Autodesk Inventor part; units mm, degrees
ref_plane "YZ Plane" through (0, 0, 0) normal (1, 0, 0) x (0, 1, 0)
ref_plane "XZ Plane" through (0, 0, 0) normal (0, 1, 0) x (-1, 0, 0)
ref_plane "XY Plane" through (0, 0, 0) normal (0, 0, 1) x (1, 0, 0)
ref_plane "Work Plane3" through (0, 0, 0) normal (0, 0, 1) x (1, 0, 0)
sketch "Sketch2" plane through (0, 0, 0) normal (0, 0, 1) x (1, 0, 0)
  arc A0 (-7.5753, -9.9544) -> (-9.0817, -9.6822) centre (-8, -8) ccw construction
  arc A1 (-9.9544, 7.5753) -> (-9.6822, 9.0817) centre (-8, 8) ccw construction
  line L0 (-8, 8) -> (-8, -8) construction
  line L1 (-3.2375, 8) -> (-3.2375, -8)
  line L2 (-12.7625, 8) -> (-12.7625, -3.2375)
  arc A2 (-3.2375, 8) -> (-12.7625, 8) centre (-8, 8) ccw
  arc A3 (-3.2375, 8) -> (-12.7625, 8) centre (-8, 8) ccw construction
  arc A4 (-8, -12.7625) -> (-3.2375, -8) centre (-8, -8) ccw
  line L3 (-76.8525, -130.4672) -> (11.0654, 135.3719) construction
  line L4 (-12.7625, -3.2375) -> (-34.7753, -3.2375)
  line L5 (-67.8092, -133.458) -> (20.1087, 132.3811) construction
  line L6 (-8, -12.7625) -> (-27.893, -12.7625)
  arc A5 (1.9836, 0.2558) -> (1.5702, -1.2387) centre (0, 0) ccw construction
  circle A6 centre (0, 0) radius 115.8748 construction
  line L7 (-34.7753, -3.2375) -> (-65.3505, -95.6884)
  line L8 (-65.3505, -95.6884) -> (-56.2232, -98.425)
  line L9 (-27.893, -12.7625) -> (-56.2232, -98.425)
  line L10 (-27.893, -12.7625) -> (-36.9363, -9.7717) construction
  line L11 (-60.7868, -97.0567) -> (-32.4146, -11.2671) construction
  circle A7 centre (-35.4852, -20.5515) radius 1.9685
  circle A8 centre (-38.5557, -29.836) radius 1.9685
  circle A9 centre (-41.6262, -39.1204) radius 1.9685
  circle A10 centre (-44.6968, -48.4048) radius 1.9685
  circle A11 centre (-47.7673, -57.6893) radius 1.9685
  circle A12 centre (-50.8378, -66.9737) radius 1.9685
  circle A13 centre (-53.9084, -76.2581) radius 1.9685
  circle A14 centre (-56.9789, -85.5426) radius 1.9685
  circle A15 centre (-8, -8) radius 2.2479
  circle A16 centre (-8, 8) radius 2.2479
  point P0 (0, 0)
  dimension "d6" = 231.7496
  dimension "d0" = 4.7625
  dimension "d1" = 4.7625
  dimension "d2" = 4.7625
  dimension "d3" = 4.7625
  dimension "d4" = 9.525
  dimension "d5" = 9.525
  dimension "d7" = 3.937
  dimension "d8" = 9.779
  dimension "d11" = 9.779
  dimension "d16" = 4.4958
  dimension "d17" = 4.4958
extrude "Extrusion1" add sketch "Sketch2" along normal blind 3.175
properties part number "CollectorArmZ"
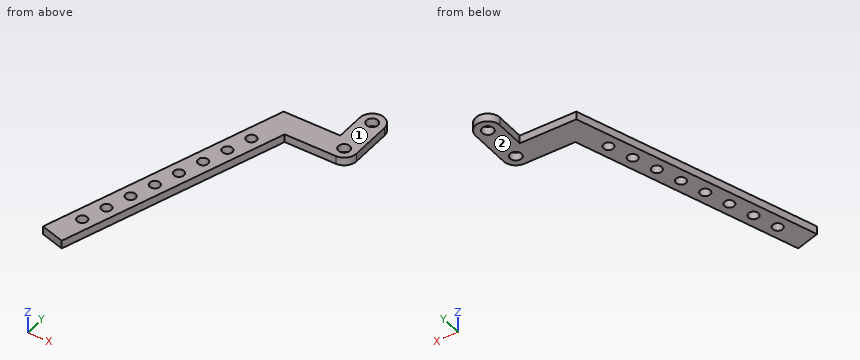
Can you work these out from the model? Positions are in its coordinate system, mm. Face numbers are marked on the shaded views. Coordinates: 2 decimals unless noted, no trailing zeros. Loops run counter-clockwise (first coordinate to the right, second up) from the corner with the lowest first, then second, coordinate; pieces in that order, holes last. Notation, with made-up numbers: M 41.5,6.5 L 65.5,6.5 A22 ccw 65.5,44.5 Z; hole C -24.75,76.25 d10. An arc over 180 degrees is marked long. Return JSON: item names as keys, results as strings. Group by question number.
Item 1: Imagine slicing it at C-C (x = -60.5). Please give me the cut outline in (y, z) (3 decimals), and give its area (3 significant figures).
Item 2: Thinking about a two-plate mould opening in Z: for the marked faces 1 and 2, which applies, released by +Z, released by -Z, zero draft, split by the parting line, or undercut?
Item 3: Imagine slicing it at B-B (y = 3). Please give me the cut outline in (x, z) (1 decimal).
Item 4: I'm going to push flat-ended pins straight in: pin 1 Ø1.5 at (y, z) = (-25.5, 2) entering from +X; pin 2 Ø1.5 at (y, z) = (-9.5, 1) entering from -X. Where does each tip first touch, or does it pass through?
Item 5: Imagine slicing it at A-A (z = 0.8). Give the number of separate pieces and of enclosed holes in the cut face, and give its area (3 significant figures).
Item 6: If I drill on L1, parallel to Y at x = -8, z = 2; L2, parallel to Y at x = -10, z = 0.2; L3, parallel to Y at x = -26.5, z = 0.35, over which ranges is the centre line in solid material (lowest first)? Write a range as from..to.
Verdict:
{
 "1": {"outline": "M -97.143,0 L -81.022,0 L -81.022,3.175 L -97.143,3.175 Z", "area": "51.2 mm^2"},
 "2": {"face 1": "released by +Z", "face 2": "released by -Z"},
 "3": {"outline": "M -12.8,0 L -3.2,0 L -3.2,3.2 L -12.8,3.2 Z"},
 "4": {"pin 1": "stops at x = -31.86", "pin 2": "stops at x = -37.09"},
 "5": {"separate pieces": "1", "enclosed holes": "10", "area": "1,170 mm^2"},
 "6": {"L1": "y = -12.76..-10.25, -5.75..5.75, 10.25..12.76", "L2": "y = -12.76..-9.03, -6.97..6.97, 9.03..12.32", "L3": "y = -12.76..-3.24"}
}
